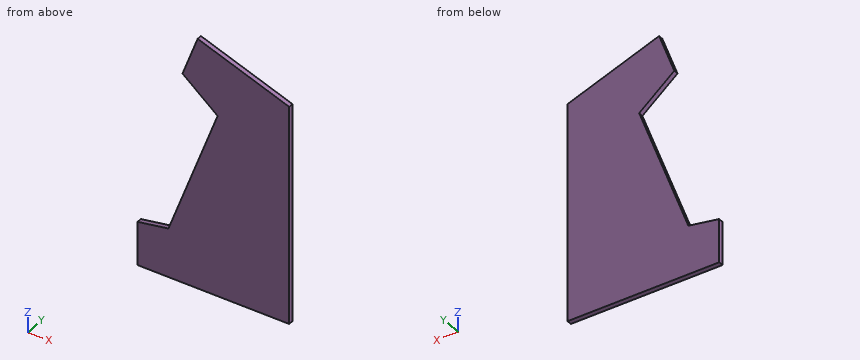
```python
from build123d import *

# Parameters (mm, degrees)
PAD_DEPTH = 13


with BuildPart() as part:
    # Sketch → Pad (new body)
    with BuildSketch(Plane.XZ):
        Polygon((0, 0), (280, 0), (280, 445.460485), (280, 602.368169), (32.503594, 692.449494), (-8.538824, 579.68638), (86.427706, 500), (-46.523657, 134.719131), (-130, 120), (-130, 0), align=None)
    extrude(amount=-PAD_DEPTH)


solid = part.part
```
Input: part model. Units: mm. Frame: model coordinates. Coordinates: 2 decimals unless noted, no trailing zeros. Write each loop counter-clockwise with the first axis right and the second up, starting at its lowest first coordinate (ties: lowest second). Pieces come first, ordered by that corner, then holes.
1) Pin query (flat end, axial travel): pin 1 Ø6 at (x, y) = (141, 5) entering from +Z; pin 2 Ø2 at (y, z) = (5.5, 355) entering from -X. Return the tip coordinate at first contact, or that it passes through.
2) Material intervals for line 1 along Z through (x, y) = (-77, 11.25); line 2 along X through (y, z) = (4.5, 397.5); line 3 along Z through (x, y) = (130, 5.5), sorted ascending.
3) Section B-B on y = 6.25. Output: boundary loops of the cut face in (x, z).
4) Section D-D on x = -2. Output: boundary loops of the cut face in (y, z).
5) Section A-A on x = 63.5. Output: boundary loops of the cut face in (y, z).
6) Section C-C on z = 200.5. Output: boundary loops of the cut face in (x, y), and give its area (3 significant figures).
Check result:
1. pin 1: stops at z = 654.05
1. pin 2: stops at x = 33.29
2. line 1: z = 0 to 129.35
2. line 2: x = 49.12 to 280
2. line 3: z = 0 to 656.96
3. outline: (-130, 0) - (280, 0) - (280, 602.37) - (32.5, 692.45) - (-8.54, 579.69) - (86.43, 500) - (-46.52, 134.72) - (-130, 120) - close
4. outline: (0, 0) - (13, 0) - (13, 257.05) - (0, 257.05) - close; (0, 574.2) - (13, 574.2) - (13, 597.65) - (0, 597.65) - close
5. outline: (0, 0) - (13, 0) - (13, 437.01) - (0, 437.01) - close; (0, 519.24) - (13, 519.24) - (13, 681.17) - (0, 681.17) - close
6. outline: (-22.58, 0) - (280, 0) - (280, 13) - (-22.58, 13) - close
6. area: 3,930 mm2
